Geometry: final body of the model. Coordinates: model frame, mm. A direction names the side the tool comes from. Give positions to 0.01 mm unless a question says otherwise; leave off trailing zeros. Loops run counter-clockwise (first coordinate to the right, second up) from the corner with the lowest first, then second, coordinate; pieces in that order, holes last. Notation, with made-up numbers: (26, 43.5) -> (38, 43.5) arc R16 cw to (38, 60.5) -> close; hole circle Ø11 at (63.25, -23.75). An arc over 180 degrees is marked (long way). One line per question, with ' | ' between items. Start each with the question number.
Item 1: Set-up query: faces 4 (the flat face through (212.898, -70, -169)), 5 (the cylindrical face through (-11.2, 62.04, 97.31)). Return all of +Z, -Z, +X, -X, +Y, -Y with unobstructed straight access to the full face (end or side cutting, diameter ignored); none if empty.
Item 2: Section B-B on x = 154.5. Return loops of the section in (y, z).
Item 3: Material intervals for line 1 along Z through (x, y) = (113.5, 0); line 2 along Y through (x, z) = (-2, 0), sorted ascending. Write a range as [from, to].
Item 4: Pin query (flat end, axial travel): P1, Ø6, axis at x = 80, y = 122, coming from the -Z side; P2, Ø4, axis at x = 180, z = 61.5, coming from the -Y side; P3, Ø12, axis at x = 76.5, y = 111, coming from the +Z side. Return the tip coordinate at first contact, or that it passes through.
Item 5: Section C-C on x = 32. Return loops of the section in (y, z), then the cut area to 3 significant figures.
Item 6: Mould query, pull axis Z, two halves, no side actions, for faces 1 (the cylindrical face through (136.783, -39.413, -177.485)), 2 (the flat face through (-28.978, 51, -93)), 3 (the cylindrical face through (133.796, -41.472, -186.762)). Classes: released by +Z, released by -Z, zero draft, split by the parting line, or undercut.
Item 7: Section A-A on y = 0. Return loops of the section in (x, z), then the cut area to 3 significant figures.
from build123d import *

# Parameters (mm, degrees)
SKETCH81_W          = 180
SKETCH81_H          = 433.466768404
EXTRUDE1_DEPTH      = 189
EXTRUDE1_DEPTH_BACK = 4.64655855
BOSS_EXTRUDE1_DEPTH = 25.4
BOSS_EXTRUDE2_DEPTH = 25.4
SCALE1_SCALE        = 0.99764556
SKETCH86_W          = 340
SKETCH86_H          = 440
CUT_EXTRUDE3_DEPTH  = 25.841374544
REVOLVE1_ANGLE      = 180


with BuildPart() as part:
    # Sketch1 → Revolve-Thin1 (revolve)
    with BuildSketch(Plane.XY, mode=Mode.PRIVATE) as revolve_thin1_sk:
        with BuildLine():
            Line((188, 191.7625), (57.01221252, 191.7625))
            ThreePointArc((57.01221252, 191.7625), (53.572316909, 190.822243935), (51.088985501, 188.262941607))
            Line((51.088985501, 188.262941607), (13.030109919, 119.174558393))
            ThreePointArc((13.030109919, 119.174558393), (10.546778511, 116.615256065), (7.1068829, 115.675))
            Line((7.1068829, 115.675), (-3.64655855, 115.675))
            Line((-3.64655855, 115.675), (-3.64655855, 106.15))
            Line((-3.64655855, 106.15), (7.1068829, 106.15))
            ThreePointArc((7.1068829, 106.15), (15.391881017, 108.41460934), (21.372991598, 114.578696092))
            Line((21.372991598, 114.578696092), (58.64435156, 182.2375))
            Line((58.64435156, 182.2375), (188, 182.2375))
            Line((188, 182.2375), (188, 191.7625))
        make_face()
    revolve(revolve_thin1_sk.sketch.rotate(Axis((0, 0, 0), (1, 0, 0)), 270), axis=Axis((0, 0, 0), (1, 0, 0)))  # turned: the seam where the file's is

    # Sketch81 → Extrude1 (cut, two sides)
    with BuildSketch(Plane(origin=(0, 0, 0), x_dir=(0, 0, -1), z_dir=(1, 0, 0))) as extrude1_sk:
        with Locations((-114.9, 1.572115024)):
            Rectangle(SKETCH81_W, SKETCH81_H)
    extrude(amount=EXTRUDE1_DEPTH, mode=Mode.SUBTRACT)
    extrude(extrude1_sk.sketch, amount=-EXTRUDE1_DEPTH_BACK, mode=Mode.SUBTRACT)

    # Sketch82 → Boss-Extrude1 (add)
    with BuildSketch(Plane.ZY.offset(3.64655855)):
        with BuildLine():
            Line((24.9, 103.188238186), (24.9, 112.963249002))
            ThreePointArc((24.9, 112.963249002), (-115.675, 0), (24.9, -112.963249002))
            Line((24.9, -112.963249002), (24.9, -103.188238186))
            ThreePointArc((24.9, -103.188238186), (-106.15, 0), (24.9, 103.188238186))
        make_face()
    extrude(amount=BOSS_EXTRUDE1_DEPTH)

    # Sketch83 → Boss-Extrude2 (add)
    with BuildSketch(Plane(origin=(188, 0, 0), x_dir=(0, 0, -1), z_dir=(1, 0, 0))):
        with BuildLine():
            Line((-24.9, -180.528381166), (-24.9, -190.139018632))
            ThreePointArc((-24.9, -190.139018632), (191.7625, 0), (-24.9, 190.139018632))
            Line((-24.9, 190.139018632), (-24.9, 180.528381166))
            ThreePointArc((-24.9, 180.528381166), (182.2375, 0), (-24.9, -180.528381166))
        make_face()
    extrude(amount=BOSS_EXTRUDE2_DEPTH)


with BuildPart() as part_1:
    # Scale1: scaled about (0, 0, 0)
    add(part.part.scale(SCALE1_SCALE))

    # Sketch86 → Cut-Extrude3 (cut, through all)
    with BuildSketch(Plane.XY):
        with Locations((100, 0)):
            Rectangle(SKETCH86_W, SKETCH86_H)
    extrude(amount=CUT_EXTRUDE3_DEPTH, mode=Mode.SUBTRACT)

    # Sketch87 → Revolve1 (revolve)
    with BuildSketch(Plane.XY):
        with BuildLine():
            Line((58.506276953, 181.808432741), (212.897562504, 181.808432741))
            Line((212.897562504, 181.808432741), (212.897562504, 191.3110067))
            Line((212.897562504, 191.3110067), (56.877980686, 191.3110067))
            ThreePointArc((56.877980686, 191.3110067), (53.446184103, 190.372964411), (50.96869955, 187.819687807))
            Line((50.96869955, 187.819687807), (12.999431307, 118.893969046))
            ThreePointArc((12.999431307, 118.893969046), (10.521946754, 116.340692442), (7.090150171, 115.402650153))
            Line((7.090150171, 115.402650153), (-28.978170171, 115.402650153))
            Line((-28.978170171, 115.402650153), (-28.978170171, 105.900076194))
            Line((-28.978170171, 105.900076194), (7.090150171, 105.900076194))
            ThreePointArc((7.090150171, 105.900076194), (15.355641757, 108.159353648), (21.322670172, 114.308927427))
            Line((21.322670172, 114.308927427), (58.506276953, 181.808432741))
        make_face()
    revolve(axis=Axis((224.991349138, 0, 0), (1, 0, 0)), revolution_arc=REVOLVE1_ANGLE)


solid = part_1.part
Result sheet:
1) face 4: +Z, -Z, +X, +Y, -Y | face 5: -X
2) outline: circle Ø382.62 at (0, 0); hole circle Ø363.62 at (0, 0)
3) line 1: z = [-191.31, -181.81], [181.81, 191.31] | line 2: y = [-115.4, -105.9], [105.9, 115.4]
4) P1: stops at z = -149.8 | P2: stops at y = -181.82 | P3: stops at z = 159.92
5) outline: circle Ø306.77 at (0, 0); hole circle Ø267.38 at (0, 0) | area: 17,800 mm²
6) face 1: undercut | face 2: zero draft | face 3: split by the parting line
7) outline: (-28.98, -115.4) -> (7.09, -115.4) arc R6.75 cw to (13, -118.89) -> (50.97, -187.82) arc R6.75 ccw to (56.88, -191.31) -> (212.9, -191.31) -> (212.9, -181.81) -> (58.51, -181.81) -> (21.32, -114.31) arc R16.25 ccw to (7.09, -105.9) -> (-28.98, -105.9) -> close; (-28.98, 105.9) -> (7.09, 105.9) arc R16.25 ccw to (21.32, 114.31) -> (58.51, 181.81) -> (212.9, 181.81) -> (212.9, 191.31) -> (56.88, 191.31) arc R6.75 ccw to (50.97, 187.82) -> (13, 118.89) arc R6.75 cw to (7.09, 115.4) -> (-28.98, 115.4) -> close | area: 5,420 mm²
